Build history of the part. All positions in model axes, mm. Round coordinates to 2 decimals unless told otherwise and drop trailing zeros. Write each loop counter-clockwise with the first axis right and the second up, starting at its lowest first coordinate (ties: lowest second). Pieces come first, ordered by that corner, then holes. Notation, with made-up numbers: (65.5, -4) -> (82.5, -4) arc R21 cw to (82.5, 2) -> close; hole circle Ø4 at (-25.5, 15.25). An arc over 180 degrees is marked (long way). Return JSON: item names as keys, results as strings.
from build123d import *

# Parameters (mm, degrees)
F0_R     = 45
F1_DEPTH = 70
F4_R     = 2
F5_R     = 15
F6_DEPTH = 88.4901


with BuildPart() as f1:
    # F0 (on Top) → F1 (new body)
    with BuildSketch(Plane.XY):
        Circle(F0_R)
    extrude(amount=F1_DEPTH)

    # F2 (on Front) → F3 (revolve, cut)
    with BuildSketch(Plane.XZ):
        with BuildLine():
            Line((0, 70), (0, 66))
            add(Edge.make_bspline(
                [(0, 66), (45, 66), (45, 70)],
                knots=[4.7123889804, 4.7123889804, 4.7123889804, 6.2831853072, 6.2831853072, 6.2831853072], degree=2, weights=[1, 0.7071067812, 1]))
            Line((45, 70), (0, 70))
        make_face()
    revolve(axis=Axis((0, 0, 35), (0, 0, 1)), mode=Mode.SUBTRACT)

    # F4
    f4_edges = [f1.edges().sort_by_distance(p)[0] for p in [
        (-45, 0, 70),
    ]]
    fillet(f4_edges, radius=F4_R)

    # F5 (on Top) → F6 (cut)
    with BuildSketch(Plane.XY):
        Circle(F5_R)
    extrude(amount=F6_DEPTH, mode=Mode.SUBTRACT)


solid = f1.part
Q1. Two-plate mould, pull along X, no slides. Class faces 1 (the cylindrical face through (-14.985, 0.66, 32.651)), 2 (the cylindrical face through (-9.76, -43.93, 32.91)), 3 (the flat face through (-11, 11, 0)): +X half, -X half, draft (parallel to the pull), parting line (faces both ways), or undercut.
Verdict:
{"face 1": "undercut", "face 2": "parting line", "face 3": "draft"}
Q2. Pin check, flat tips, straight feed: pin 1 Ø3 at (x, y) = (11, 30.5) entering from +Z; pin 2 Ø8 at (x, z) = (3, 40) entering from -Y; pin 3 Ø4 at (y, z) = (-33.5, 18) entering from -X. Stop position of each tip, or through.
Verdict:
{"pin 1": "stops at z = 67.37", "pin 2": "stops at y = -45", "pin 3": "stops at x = -32.14"}
Q3. Wall check: L1, parallel to X at y = 0, z = 33; L2, parallel to Z at x = -6, y = 25.5. Give the ranges that are in metal, low to high.
Verdict:
{"L1": "x = -45 to -15, 15 to 45", "L2": "z = 0 to 66.75"}
Q4. Saw through at A-A on z = 29. List the corners of the cut face in (x, y), then the cut area to 3 significant figures.
Verdict:
{"outline": "circle Ø90 at (0, 0); hole circle Ø30 at (0, 0)", "area": "5,650 mm²"}
